Read the model definition and answer for the solid it produces. Units are mm, in the model's axes. Face numbers are marked on the shaded views. A direction names the side the tool comes from. Coordinates: 2 decimals unless noted, no trailing zeros. Order: outer loops, then holes, each group sorted by start corner. A loop starts at its lowest first (then second) coordinate and runs counter-clockwise, first axis right, second up. Notation, with made-up numbers: (0, 81.25) -> (10, 81.25) arc R23 ccw to (10, 108.25) -> close; hole circle Ø4 at (35, 67). An arc over 180 degrees is marked (long way). Return JSON: item names as keys, results as strings. Group by question number.
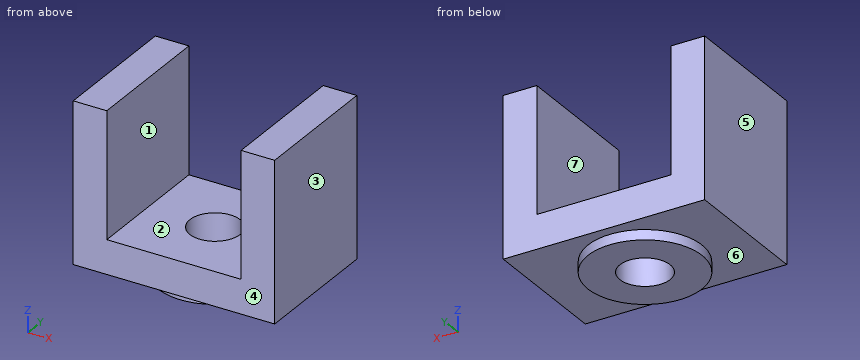
```python
from build123d import *

# Parameters (mm, degrees)
F0_W     = 60
F0_H     = 40
F1_DEPTH = 50.5
F2_W     = 60
F2_H     = 3
F3_DEPTH = 40.001
F4_R     = 17
F5_DEPTH = 3
F6_W     = 40
F6_H     = 37.407568
F7_DEPTH = 40.001
F8_R     = 7.5
F9_DEPTH = 50.501


with BuildPart() as f1:
    # F0 (on Top) → F1 (new body)
    with BuildSketch(Plane.XY):
        with Locations((30, -20)):
            Rectangle(F0_W, F0_H)
    extrude(amount=F1_DEPTH)

    # F2 (on face) → F3 (cut, through all)
    with BuildSketch(Plane.XZ.offset(40)):
        with Locations((30, 1.5)):
            Rectangle(F2_W, F2_H)
    extrude(amount=-F3_DEPTH, mode=Mode.SUBTRACT)

    # F4 (on face) → F5 (join)
    with BuildSketch(Plane(origin=(0, 0, 3), x_dir=(1, 0, 0), z_dir=(0, 0, -1))):
        with Locations((30, 20)):
            Circle(F4_R)
    extrude(amount=F5_DEPTH)

    # F6 (on face) → F7 (cut, through all)
    with BuildSketch(Plane.XZ.offset(40)):
        with Locations((30, 31.796216)):
            Rectangle(F6_W, F6_H)
    extrude(amount=-F7_DEPTH, mode=Mode.SUBTRACT)

    # F8 (on face) → F9 (cut, through all)
    with BuildSketch(Plane(origin=(0, 0, 0), x_dir=(1, 0, 0), z_dir=(0, 0, -1))):
        with Locations((30, 20)):
            Circle(F8_R)
    extrude(amount=-F9_DEPTH, mode=Mode.SUBTRACT)


solid = f1.part
```
1. Find section B-B on x = 30. Determine the outline of the cut face in (y, z).
2. Find section A-A on y = -20. Determine the outline of the cut face in (x, z).
3. Given pin 1 (1 mm diameter, centred on y = -31.5, z = 16, fed in from -X); pin 2 (12 mm diameter, centred on x = 36.5, y = -17, fed in from +Z), each flat-ended and moving along its own axis, determine where each tip first touches the part or whether it passes through.
4. Find section C-C on z = 40. Determine the outline of the cut face in (x, y).
5. Straight lines are drawn through the part: L1, parallel to X at y = -4, z = 43; L2, parallel to X at y = -20, z = 5.5; L3, parallel to Y at x = 30.5, z = 8. For each, find the intervals that lie inside material, in ascending order.
6. Find section D-D on x = 45. Determine the outline of the cut face in (y, z).
7. For a pull along X with two mould halves and no side action, classify the marked faces 1, 2, 3 and 4 as released by +X, released by -X, zero draft, split by the parting line, or undercut.
8. Which of the six approach directions +Z, -Z, +X, -X, +Y, -Y give full straight-line access (tool end or side, diameter ignored) to the marked faces 5, 6 and 7?
Result:
{
 "1": {"outline": "(-40, 3) -> (-37, 3) -> (-37, 0) -> (-27.5, 0) -> (-27.5, 13.09) -> (-40, 13.09) -> close; (-12.5, 0) -> (-3, 0) -> (-3, 3) -> (0, 3) -> (0, 13.09) -> (-12.5, 13.09) -> close"},
 "2": {"outline": "(0, 3) -> (13, 3) -> (13, 0) -> (22.5, 0) -> (22.5, 13.09) -> (10, 13.09) -> (10, 50.5) -> (0, 50.5) -> close; (37.5, 0) -> (47, 0) -> (47, 3) -> (60, 3) -> (60, 50.5) -> (50, 50.5) -> (50, 13.09) -> (37.5, 13.09) -> close"},
 "3": {"pin 1": "x = 0", "pin 2": "z = 13.09"},
 "4": {"outline": "(0, -40) -> (10, -40) -> (10, 0) -> (0, 0) -> close; (50, -40) -> (60, -40) -> (60, 0) -> (50, 0) -> close"},
 "5": {"L1": "0 to 10, 50 to 60", "L2": "0 to 22.5, 37.5 to 60", "L3": "-40 to -27.48, -12.52 to 0"},
 "6": {"outline": "(-40, 3) -> (-28, 3) -> (-28, 0) -> (-12, 0) -> (-12, 3) -> (0, 3) -> (0, 13.09) -> (-40, 13.09) -> close"},
 "7": {"face 1": "undercut", "face 2": "undercut", "face 3": "released by +X", "face 4": "zero draft"},
 "8": {"face 5": "+Z, -Z, -X, +Y, -Y", "face 6": "-Z", "face 7": "+Z, +Y, -Y"}
}
